Model file for the job. Use its own axes, mm. Face numbers are marked on the shaded views. A direction names the side the tool comes from. Round coordinates to 2 decimals unless told otherwise and drop trailing zeros. Order: outer loops, then holes, each group sorted by start corner. A loop starts at its lowest first (then second) coordinate and runs counter-clockwise, first axis right, second up. Notation, with made-up numbers: (32.5, 0) -> (62.5, 0) arc R8 cw to (62.5, 12) -> close; hole circle Ø10 at (-0.75, 41.5). An arc over 180 degrees is marked (long way). Answer as CSV lines item,"result".
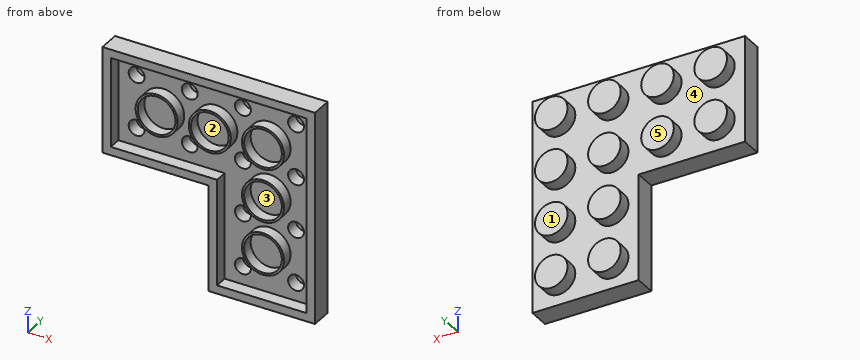
```python
from build123d import *

# Parameters (mm, degrees)
BOSS_EXTRUDE1_DEPTH = 3.17
SKETCH3_R           = 2.44
BOSS_EXTRUDE2_DEPTH = 1.95
SHELL1_T            = -1.25
SKETCH4_R           = 3.15
SKETCH4_R_2         = 2.825
BOSS_EXTRUDE3_DEPTH = 1.65


with BuildPart() as part:
    # Sketch2 → Boss-Extrude1 (new body)
    with BuildSketch(Plane(origin=(0, 0, 0), x_dir=(1, 0, 0), z_dir=(0, 1, 0))):
        Polygon((0, 0), (-15.91, 0), (-15.91, -15.91), (15.91, -15.91), (15.91, 15.91), (0, 15.91), align=None)
    extrude(amount=-BOSS_EXTRUDE1_DEPTH)

    # Sketch3 → Boss-Extrude2 (add)
    with BuildSketch(Plane(origin=(0, 0, 0), x_dir=(1, 0, 0), z_dir=(0, 1, 0))):
        with Locations(Location((11.9325, 11.9325, 0), (0, 0, 90))):
            Circle(SKETCH3_R)
        with Locations(Location((11.9325, 3.9725, 0), (0, 0, 90))):
            Circle(SKETCH3_R)
        with Locations(Location((11.9325, -3.9875, 0), (0, 0, 90))):
            Circle(SKETCH3_R)
        with Locations(Location((11.9325, -11.9475, 0), (0, 0, 90))):
            Circle(SKETCH3_R)
        with Locations(Location((3.9775, 3.9725, 0), (0, 0, 90))):
            Circle(SKETCH3_R)
        with Locations(Location((3.9775, -3.9875, 0), (0, 0, 90))):
            Circle(SKETCH3_R)
        with Locations(Location((3.9775, -11.9475, 0), (0, 0, 90))):
            Circle(SKETCH3_R)
        with Locations(Location((3.9775, 11.9325, 0), (0, 0, 90))):
            Circle(SKETCH3_R)
        with Locations(Location((-11.93, -3.98, 0), (0, 0, 90))):
            Circle(SKETCH3_R)
        with Locations(Location((-3.975, -3.98, 0), (0, 0, 90))):
            Circle(SKETCH3_R)
        with Locations(Location((-3.975, -11.935, 0), (0, 0, 90))):
            Circle(SKETCH3_R)
        with Locations(Location((-11.93, -11.935, 0), (0, 0, 90))):
            Circle(SKETCH3_R)
    extrude(amount=BOSS_EXTRUDE2_DEPTH)

    # Shell1
    shell1_openings = [part.faces().sort_by_distance(p)[0] for p in [
        (2.651666667, -3.17, 2.651666667),
    ]]
    offset(amount=SHELL1_T, openings=shell1_openings, kind=Kind.INTERSECTION)

    # Sketch4 → Boss-Extrude3 (add)
    # profile 1 of 5: a face of its own
    with BuildSketch(Plane.XZ.offset(1.25)):
        with Locations(Location((-7.955, 7.955, 0), (0, 0, 270))):
            Circle(SKETCH4_R)
        with Locations(Location((-7.955, 7.955, 0), (0, 0, 270))):
            Circle(SKETCH4_R_2, mode=Mode.SUBTRACT)
    # profile 2 of 5: a face of its own
    with BuildSketch(Plane.XZ.offset(1.25)):
        with Locations(Location((0.005, 7.955, 0), (0, 0, 270))):
            Circle(SKETCH4_R)
        with Locations(Location((0.005, 7.955, 0), (0, 0, 270))):
            Circle(SKETCH4_R_2, mode=Mode.SUBTRACT)
    # profile 3 of 5: a face of its own
    with BuildSketch(Plane.XZ.offset(1.25)):
        with Locations(Location((7.965, 7.955, 0), (0, 0, 270))):
            Circle(SKETCH4_R)
        with Locations(Location((7.965, 7.955, 0), (0, 0, 270))):
            Circle(SKETCH4_R_2, mode=Mode.SUBTRACT)
    # profile 4 of 5: a face of its own
    with BuildSketch(Plane.XZ.offset(1.25)):
        with Locations(Location((7.965, -0.005, 0), (0, 0, 270))):
            Circle(SKETCH4_R)
        with Locations(Location((7.965, -0.005, 0), (0, 0, 270))):
            Circle(SKETCH4_R_2, mode=Mode.SUBTRACT)
    # profile 5 of 5: a face of its own
    with BuildSketch(Plane.XZ.offset(1.25)):
        with Locations(Location((7.965, -7.965, 0), (0, 0, 270))):
            Circle(SKETCH4_R)
        with Locations(Location((7.965, -7.965, 0), (0, 0, 270))):
            Circle(SKETCH4_R_2, mode=Mode.SUBTRACT)
    extrude(amount=BOSS_EXTRUDE3_DEPTH)


solid = part.part
```
Q1. Saw through at C-C (x = -7). Write the cut outline in (y, z).
Checks:
outline,"(-3.17, 0) -> (0, 0) -> (0, 15.91) -> (-3.17, 15.91) -> (-3.17, 14.66) -> (-1.25, 14.66) -> (-1.25, 10.96) -> (-2.9, 10.96) -> (-2.9, 10.61) -> (-1.25, 10.61) -> (-1.25, 5.3) -> (-2.9, 5.3) -> (-2.9, 4.95) -> (-1.25, 4.95) -> (-1.25, 1.25) -> (-3.17, 1.25) -> close"
Q2. Flat gauge pins, fed straight in: pin 1 (4 mm diameter, centred on x = 5.5, z = -3.5, fed in from -Y); pin 2 (8 mm diameter, centred on x = 11, z = -6.5, fed in from +Y); pin 3 (0.7 mm diameter, centred on x = 11.5, z = -11.5, fed in from -Y); pin 4 (1 mm diameter, centred on y = -2, z = -5, fed in from -X). Where does each tip first touch, or does it go through?
Checks:
pin 1,"y = -2.9"
pin 2,"y = 1.95"
pin 3,"y = 0.7"
pin 4,"x = 0"
Q3. Mould opens along X. For the marked faces 3, 4 and 5 say: +X half, -X half, draft (parallel to the pull), parting line (faces both ways), or undercut.
Checks:
face 3,"undercut"
face 4,"undercut"
face 5,"draft"
Q4. Wall check: L1, parallel to X at y = -0.35, z = 3.98 (3 decimals); L2, parallel to X at y = -0.95, z = 11; L3, parallel to X at y = -1.8, z = 13.5. Give the ranges that are in metal, low to high. Write a range as [from, to].
Checks:
L1,"[-15.91, -13.12], [-10.74, -5.165], [-2.785, 2.788], [5.167, 10.743], [13.122, 15.91]"
L2,"[-15.91, -12.67], [-11.19, -4.71], [-3.24, 3.26], [4.7, 11.21], [12.65, 15.91]"
L3,"[-15.91, -14.66], [14.66, 15.91]"
Q5. Tool access for the marked faces 1 and 2: list every direction of +Z, -Z, +X, -X, +Y, -Y with a clear straight run to the whole face (end or side of a thin tool).
Checks:
face 1,"+Z, -Z, +X, -X, +Y"
face 2,"-Y"
Q6. Saw through at B-B (z = -7). Write the cut outline in (x, y).
Checks:
outline,"(0, -3.17) -> (1.25, -3.17) -> (1.25, -1.25) -> (4.97, -1.25) -> (4.97, -2.9) -> (5.31, -2.9) -> (5.31, -1.25) -> (10.62, -1.25) -> (10.62, -2.9) -> (10.96, -2.9) -> (10.96, -1.25) -> (14.66, -1.25) -> (14.66, -3.17) -> (15.91, -3.17) -> (15.91, 0) -> (0, 0) -> close"
Q7. Saw through at A-A (x = -11.93). Write the cut outline in (y, z) (3 decimals).
Checks:
outline,"(-3.17, 0) -> (0, 0) -> (0, 1.54) -> (1.95, 1.54) -> (1.95, 6.42) -> (0, 6.42) -> (0, 9.495) -> (1.95, 9.495) -> (1.95, 14.375) -> (0, 14.375) -> (0, 15.91) -> (-3.17, 15.91) -> (-3.17, 14.66) -> (-1.25, 14.66) -> (-1.25, 13.125) -> (0.7, 13.125) -> (0.7, 10.745) -> (-1.25, 10.745) -> (-1.25, 5.17) -> (0.7, 5.17) -> (0.7, 2.79) -> (-1.25, 2.79) -> (-1.25, 1.25) -> (-3.17, 1.25) -> close"
